from build123d import *

# Parameters (mm, degrees)
SKETCH1_W               = 540
SKETCH1_H               = 86.2
BOSS_EXTRUDE1_DEPTH     = 3.175
SKETCH2_W               = 25.75
SKETCH2_H               = 40
CUT_EXTRUDE1_DEPTH      = 274.436812856
F_1_4_CLEARANCE_HOLE1_D = 6.5278
DRAFT1_ANGLE            = 10
FILLET1_R               = 12
CHAMFER1_SIZE           = 6
SKETCH5_R               = 3.3
CUT_EXTRUDE2_DEPTH      = 287.180297864
BOSS_EXTRUDE2_DEPTH     = 3.175
FILLET2_R               = 10
SKETCH8_W               = 15.55
SKETCH8_H               = 13
BOSS_EXTRUDE3_DEPTH     = 3.175
SKETCH9_R               = 1.5
CUT_EXTRUDE3_DEPTH      = 289.424622537
FILLET3_R               = 1
SKETCH10_W              = 5.1
SKETCH10_H              = 5.5
CUT_EXTRUDE4_DEPTH      = 289.424622537
SKETCH11_R              = 1.5
CUT_EXTRUDE5_DEPTH      = 289.424622537
FILLET4_R               = 1
M3X0_5_TAPPED_HOLE1_D   = 2.5


with BuildPart() as part:
    # Sketch1 → Boss-Extrude1 (new body)
    with BuildSketch(Plane.XY):
        Rectangle(SKETCH1_W, SKETCH1_H)
    extrude(amount=BOSS_EXTRUDE1_DEPTH)

    # Sketch2 → Cut-Extrude1 (cut, through all)
    with BuildSketch(Plane.XY.offset(3.175)):
        with Locations((121.62, -23.1)):
            Rectangle(SKETCH2_W, SKETCH2_H)
        with Locations((-121.62, -23.1)):
            Rectangle(SKETCH2_W, SKETCH2_H)
    extrude(amount=-CUT_EXTRUDE1_DEPTH, mode=Mode.SUBTRACT)

    # 1/4 Clearance Hole1 (through all)
    with Locations(Plane.XY.offset(3.175)):
        with Locations((-131.975, 11.9), (-111.265, 11.9), (111.265, 11.9), (131.975, 11.9)):
            Hole(F_1_4_CLEARANCE_HOLE1_D / 2)

    # Draft1
    draft1_faces = [part.faces().sort_by_distance(p)[0] for p in [
        (270, 0, 1.5875),
        (-270, 0, 1.5875),
    ]]
    draft(draft1_faces, Plane(origin=(270, 43.1, 3.175), x_dir=(1, 0, 0), z_dir=(0, 1, 0)), DRAFT1_ANGLE)

    # Fillet1
    fillet1_edges = [part.edges().sort_by_distance(p)[0] for p in [
        (-285.199385737, -43.1, 1.5875),
        (-270, 43.1, 1.5875),
        (270, 43.1, 1.5875),
        (285.199385737, -43.1, 1.5875),
    ]]
    fillet(fillet1_edges, radius=FILLET1_R)

    # Chamfer1
    chamfer1_edges = [part.edges().sort_by_distance(p)[0] for p in [
        (-134.495, -43.1, 1.5875),
        (134.495, -43.1, 1.5875),
        (108.745, -43.1, 1.5875),
        (-108.745, -43.1, 1.5875),
    ]]
    chamfer(chamfer1_edges, length=CHAMFER1_SIZE)

    # Sketch5 → Cut-Extrude2 (cut, through all)
    with BuildSketch(Plane(origin=(0, 0, 0), x_dir=(-1, 0, 0), z_dir=(0, 0, -1))):
        with Locations((-255, 24)):
            Circle(SKETCH5_R)
        with Locations((-255, 4.95)):
            Circle(SKETCH5_R)
        with Locations((-255, -8.05)):
            Circle(SKETCH5_R)
        with Locations((-255, -27.1)):
            Circle(SKETCH5_R)
        with Locations(Location((255, -27.1, 0), (0, 0, 180))):
            Circle(SKETCH5_R)
        with Locations(Location((255, -8.05, 0), (0, 0, 180))):
            Circle(SKETCH5_R)
        with Locations(Location((255, 4.95, 0), (0, 0, 180))):
            Circle(SKETCH5_R)
        with Locations(Location((255, 24, 0), (0, 0, 180))):
            Circle(SKETCH5_R)
    extrude(amount=-CUT_EXTRUDE2_DEPTH, mode=Mode.SUBTRACT)

    # Sketch6 → Boss-Extrude2 (add)
    with BuildSketch(Plane.XY.offset(3.175)):
        Polygon((-60, 43.1), (-45, 56.1), (45, 56.1), (60, 43.1), align=None)
    extrude(amount=-BOSS_EXTRUDE2_DEPTH)

    # Fillet2
    fillet2_edges = [part.edges().sort_by_distance(p)[0] for p in [
        (60, 43.1, 1.5875),
        (-60, 43.1, 1.5875),
        (-45, 56.1, 1.5875),
        (45, 56.1, 1.5875),
    ]]
    fillet(fillet2_edges, radius=FILLET2_R)

    # Sketch8 → Boss-Extrude3 (add)
    with BuildSketch(Plane.XY.offset(3.175)):
        with Locations((-121.62, -9.6)):
            Rectangle(SKETCH8_W, SKETCH8_H)
        with Locations((121.62, -9.6)):
            Rectangle(SKETCH8_W, SKETCH8_H)
    extrude(amount=-BOSS_EXTRUDE3_DEPTH)

    # Sketch9 → Cut-Extrude3 (cut, through all)
    with BuildSketch(Plane.XY.offset(3.175)):
        with Locations((-134.495, -3.1)):
            Circle(SKETCH9_R)
        with Locations((-129.395, -3.1)):
            Circle(SKETCH9_R)
        with Locations((-113.845, -3.1)):
            Circle(SKETCH9_R)
        with Locations((-108.745, -3.1)):
            Circle(SKETCH9_R)
        with Locations((113.845, -3.1)):
            Circle(SKETCH9_R)
        with Locations((108.745, -3.1)):
            Circle(SKETCH9_R)
        with Locations((134.495, -3.1)):
            Circle(SKETCH9_R)
        with Locations((129.395, -3.1)):
            Circle(SKETCH9_R)
    extrude(amount=-CUT_EXTRUDE3_DEPTH, mode=Mode.SUBTRACT)

    # Fillet3
    fillet3_edges = [part.edges().sort_by_distance(p)[0] for p in [
        (-129.395, -16.1, 1.5875),
        (-113.845, -16.1, 1.5875),
        (113.845, -16.1, 1.5875),
        (129.395, -16.1, 1.5875),
        (129.395, -4.6, 1.5875),
        (113.845, -4.6, 1.5875),
        (-113.845, -4.6, 1.5875),
        (-129.395, -4.6, 1.5875),
        (-132.995, -3.1, 1.5875),
        (-134.495, -4.6, 1.5875),
        (110.245, -3.1, 1.5875),
        (108.745, -4.6, 1.5875),
        (132.995, -3.1, 1.5875),
        (134.495, -4.6, 1.5875),
        (130.895, -3.1, 1.5875),
        (112.345, -3.1, 1.5875),
        (-108.745, -4.6, 1.5875),
        (-110.245, -3.1, 1.5875),
        (-112.345, -3.1, 1.5875),
        (-130.895, -3.1, 1.5875),
        (-140.495, -43.1, 1.5875),
        (-134.495, -37.1, 1.5875),
        (-108.745, -37.1, 1.5875),
        (102.745, -43.1, 1.5875),
        (-102.745, -43.1, 1.5875),
        (134.495, -37.1, 1.5875),
        (140.495, -43.1, 1.5875),
        (108.745, -37.1, 1.5875),
    ]]
    fillet(fillet3_edges, radius=FILLET3_R)

    # Sketch10 → Cut-Extrude4 (cut, through all)
    with BuildSketch(Plane.XY.offset(3.175)):
        with Locations((-131.945, 40.35)):
            Rectangle(SKETCH10_W, SKETCH10_H)
        with Locations((-111.295, 40.35)):
            Rectangle(SKETCH10_W, SKETCH10_H)
        with Locations((111.295, 40.35)):
            Rectangle(SKETCH10_W, SKETCH10_H)
        with Locations((131.945, 40.35)):
            Rectangle(SKETCH10_W, SKETCH10_H)
    extrude(amount=-CUT_EXTRUDE4_DEPTH, mode=Mode.SUBTRACT)

    # Sketch11 → Cut-Extrude5 (cut, through all)
    with BuildSketch(Plane.XY.offset(3.175)):
        with Locations((-134.495, 37.6)):
            Circle(SKETCH11_R)
        with Locations((-129.395, 37.6)):
            Circle(SKETCH11_R)
        with Locations((-113.845, 37.6)):
            Circle(SKETCH11_R)
        with Locations((-108.745, 37.6)):
            Circle(SKETCH11_R)
        with Locations((113.845, 37.6)):
            Circle(SKETCH11_R)
        with Locations((108.745, 37.6)):
            Circle(SKETCH11_R)
        with Locations((129.395, 37.6)):
            Circle(SKETCH11_R)
        with Locations((134.495, 37.6)):
            Circle(SKETCH11_R)
    extrude(amount=-CUT_EXTRUDE5_DEPTH, mode=Mode.SUBTRACT)

    # Fillet4
    fillet4_edges = [part.edges().sort_by_distance(p)[0] for p in [
        (-134.495, 43.1, 1.5875),
        (-129.395, 43.1, 1.5875),
        (-113.845, 43.1, 1.5875),
        (-108.745, 43.1, 1.5875),
        (108.745, 43.1, 1.5875),
        (113.845, 43.1, 1.5875),
        (129.395, 43.1, 1.5875),
        (134.495, 43.1, 1.5875),
        (-130.895, 37.6, 1.5875),
        (-132.995, 37.6, 1.5875),
        (-112.345, 37.6, 1.5875),
        (-110.245, 37.6, 1.5875),
        (108.745, 39.1, 1.5875),
        (112.345, 37.6, 1.5875),
        (129.395, 39.1, 1.5875),
        (132.995, 37.6, 1.5875),
        (-134.495, 39.1, 1.5875),
        (134.495, 39.1, 1.5875),
        (130.895, 37.6, 1.5875),
        (110.245, 37.6, 1.5875),
        (113.845, 39.1, 1.5875),
        (-108.745, 39.1, 1.5875),
        (-113.845, 39.1, 1.5875),
        (-129.395, 39.1, 1.5875),
    ]]
    fillet(fillet4_edges, radius=FILLET4_R)

    # M3x0.5 Tapped Hole1 (through all)
    with Locations(Plane(origin=(0, 0, 0), x_dir=(-1, 0, 0), z_dir=(0, 0, -1))):
        with Locations((-229.495, -23.1), (-189.495, -23.1), (-149.495, -23.1), (-80, -23.1), (-40, -23.1), (0, -23.1), (40, -23.1), (80, -23.1), (149.495, -23.1), (189.495, -23.1), (229.495, -23.1)):
            Hole(M3X0_5_TAPPED_HOLE1_D / 2)


solid = part.part
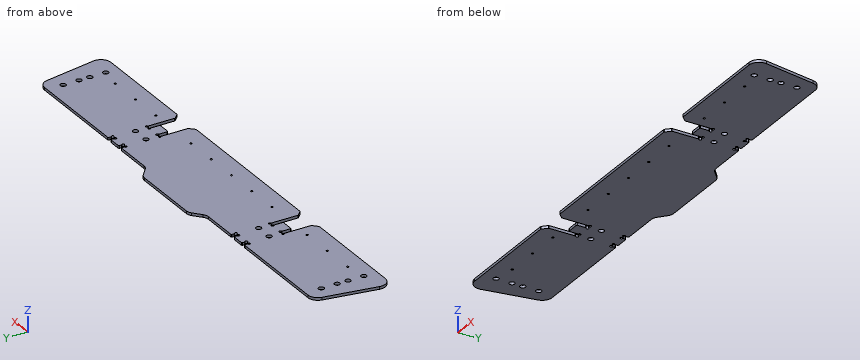
The model under review builds one solid part; all positions refer to its coordinate system, in mm. Round coordinates to 2 decimals unless told otherwise and drop trailing zeros. Write each loop counter-clockwise with the first axis right and the second up, starting at its lowest first coordinate (ties: lowest second). Pieces come first, ordered by that corner, then holes. Notation, with made-up numbers: (16.5, -10.75) -> (58.5, -10.75) arc R13 ccw to (58.5, 1.25) -> close; hole circle Ø10 at (73, -34). An arc over 180 degrees is marked (long way). Answer as a JSON object with one key per item and string values.
1. We need section A-A on z = 1.7. State how many separate pieces and enclosed holes the cut face has, and give its area (3 significant figures).
Results found:
{"separate pieces": "1", "enclosed holes": "23", "area": "46,700 mm^2"}
2. Clearance check with flat-ended pins moving along their axes: pin 1 (1 mm diameter, centred on x = -111.5, z = 2.5, fed in from -Y); pin 2 (1.8 mm diameter, centred on y = 41, z = 2, fed in from +X); pin 3 (1.1 mm diameter, centred on y = 41, z = 1.5, fed in from -X). State where each tip first meets the part, or that it passes through.
Results found:
{"pin 1": "stops at y = -3.1", "pin 2": "stops at x = 267.87", "pin 3": "stops at x = -267.45"}
3. We need section B-B on x = -197.5. State the section outline as (y, z) points (3 decimals).
Results found:
{"outline": "(-43.1, 0) -> (43.1, 0) -> (43.1, 3.175) -> (-43.1, 3.175) -> close"}
4. To check wall thickness, follow line 1 along X through (y, z) = (-33, 1.8) (3 decimals); line 2 along X through (y, z) = (-30, 3) (3 decimals); line 3 along Y through (x, z) = (-126, 1.15). State the ranges of each line that lie inside material, in increasing order.
Results found:
{"line 1": "x = -282.747 to -134.495, -108.745 to 108.745, 134.495 to 282.747", "line 2": "x = -282.848 to -256.575, -253.425 to -134.495, -108.745 to 108.745, 134.495 to 253.425, 256.575 to 282.848", "line 3": "y = -16.1 to 43.1"}
